Autodesk Inventor part; units mm, degrees
ref_plane "YZ Plane" through (0, 0, 0) normal (1, 0, 0) x (0, 1, 0)
ref_plane "XZ Plane" through (0, 0, 0) normal (0, 1, 0) x (-1, 0, 0)
ref_plane "XY Plane" through (0, 0, 0) normal (0, 0, 1) x (1, 0, 0)
sketch "Sketch1" plane through (0, 0, 0) normal (0, 0, 1) x (1, 0, 0)
  circle A0 centre (0, 0) radius 38
  circle A1 centre (0, 0) radius 33
  dimension "d0" = 76
  dimension "d1" = 66
extrude "Extrusion1" add sketch "Sketch1" along normal blind 15
sketch "Sketch2" plane through (0, 0, 0) normal (0, 0, -1) x (-1, 0, 0)
  circle A0 centre (0, 0) radius 33
  line L0 (0.0152, 1) -> (-32.9848, 1)
  line L1 (0.0152, -1) -> (-32.9848, -1)
  line L2 (0.0152, 1) -> (-12.0152, 1)
  circle A1 centre (0, 0) radius 33
  line L3 (0.0152, -1) -> (0.0152, 1)
  line L4 (-1, 0.0152) -> (-1, -32.9848)
  line L5 (1, 0.0152) -> (1, -32.9848)
  line L6 (-0.0152, -1) -> (32.9848, -1)
  line L7 (-0.0152, 1) -> (32.9848, 1)
  line L8 (1, -0.0152) -> (1, 32.9848)
  line L9 (-1, -0.0152) -> (-1, 32.9848)
  point P0 (-1, 1)
  point P1 (-1, -1)
  point P2 (1, -1)
  point P3 (1, 1)
  dimension "d12" = 2
  dimension "d17" = 66
  dimension "d18" = 33
  dimension "d19" = 33
  dimension "d22" = 360
extrude "Extrusion2" add sketch "Sketch2" against normal blind 15 contours A0 L6 L5 L8 L7 | L8 L7 L0 L9 A0 | L8 L5 L6 L3 L7 | A0 L4 L1 L6 L5 | L3 L1 L4 L9 L0 | L0 L9 L4 L1 A0
sketch "Sketch3" plane through (0, 0, 0) normal (0, 0, -1) x (-1, 0, 0)
  line L0 (0, 20) -> (-0.5, 20)
  line L1 (-0.5, 20) -> (-0.5, -20)
  line L2 (-0.5, -20) -> (0.5, -20)
  line L3 (0.5, -20) -> (0.5, 20)
  line L4 (0.5, 20) -> (0, 20)
  point P0 (0, 0)
  dimension "d27" = 20
  dimension "d29" = 40
  dimension "d30" = 1
  dimension "d31" = 40
extrude "Extrusion3" cut sketch "Sketch3" against normal blind 2
sketch "Sketch4" plane through (-1, 1, 0) normal (-1, 0, 0) x (0, 0, 1)
  point P0 (0, -1)
  point P1 (1.0253, 17.9677)
hole "Hole1" at (-1, 18.9677, 1.0253) direction (1, 0, 0) diameter 0.7 end through all
sketch "Sketch5" plane through (-1, -32.9848, 0) normal (-1, 0, 0) x (0, 0, 1)
  point P0 (0, 32.9848)
  point P1 (1.4149, 14.4794)
hole "Hole2" at (-1, -18.5055, 1.4149) direction (1, 0, 0) diameter 0.7 end through all
properties part number "SUJETADOR_MICRO"
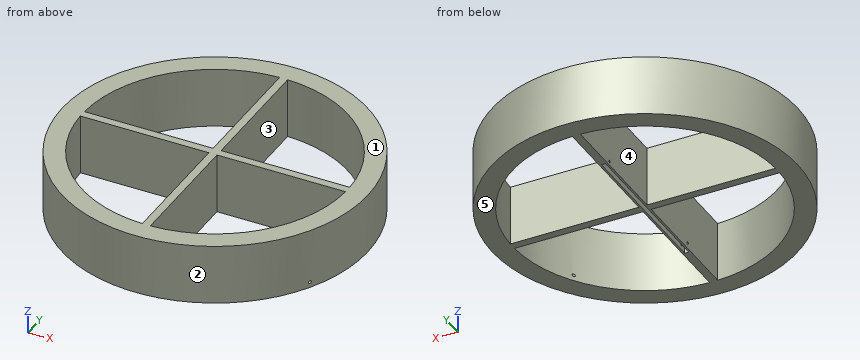
The listing builds one solid part. Answer for the finished solid, in the listing's coordinates (mm). Face numbers are marked on the shaded views. A direction names the side the tool comes from. Round coordinates to 2 decimals unless told otherwise and drop trailing zeros. Write each loop counter-clockwise with the first axis right and the second up, starting at its lowest first coordinate (ties: lowest second). Pieces come first, ordered by that corner, then holes. Notation, with made-up numbers: M -5.5,62 L 6.5,62 A22 ccw 6.5,87 Z; hole C 4.25,37.5 d2. An arc over 180 degrees is marked long. Write each question's results on one line, items separated by ' | '. Start each with the question number.
Item 1: Find section A-A on y = 30. Write down the section's boundary in (x, z).
Item 2: Find section C-C on z = 8.5. Write down the section's boundary in (x, y).
Item 3: Straight lines are drawn through the part: probe 1 along X at (y, z) = (-6, 11); probe 2 along X at (y, z) = (-12, 10). For each, find the intervals that lie inside material, in ascending order.
Item 4: Which of the six approach directions +Z, -Z, +X, -X, +Y, -Y give full straight-line access (tool end or side, diameter ignored) to the marked faces 4 and 5?
Item 5: The mould has two halves that part along X. Classify the marked faces 1, 2 and 3: +X half, -X half, draft (parallel to the pull), parting line (faces both ways), or undercut.
Item 6: Find section B-B on x = 9. Write down the section's boundary in (y, z), and give its area (3 significant figures).
Item 7: Given pin 1 Ø1 at (x, y) = (-26.5, 23.5) entering from -Z; pin 2 Ø8 at (x, z) = (-29.5, 10) entering from -Y; pin 3 Ø7.5 at (x, z) = (-17.5, 4.5) entering from -Y; pin 4 Ø0.5 at (x, z) = (0, 1) entering from -Y, each flat-ended and moving along its own axis, determine where each tip first touches the part or whether it passes through.
Answer block:
1) outline: M -23.32,0 L -13.75,0 L -13.75,15 L -23.32,15 Z; M -1,0 L 1,0 L 1,15 L -1,15 Z; M 13.75,0 L 23.32,0 L 23.32,15 L 13.75,15 Z
2) outline: C 0,0 d76; hole M -32.98,-1 A33 ccw -1,-32.98 L -1,-1 Z; hole M -32.98,1 L -1,1 L -1,32.98 A33 ccw Z; hole M 1,-32.98 A33 ccw 32.98,-1 L 1,-1 Z; hole M 1,1 L 32.98,1 A33 ccw 1,32.98 Z
3) probe 1: x = -37.52 to -32.45, -1 to 1, 32.45 to 37.52 | probe 2: x = -36.06 to -30.74, -1 to 1, 30.74 to 36.06
4) face 4: +Z, -Z | face 5: -Z, +X, -X, +Y, -Y
5) face 1: draft | face 2: parting line | face 3: undercut
6) outline: M -36.92,0 L -31.75,0 L -31.75,15 L -36.92,15 Z; M -1,0 L 1,0 L 1,15 L -1,15 Z; M 31.75,0 L 36.92,0 L 36.92,15 L 31.75,15 Z | area: 185 mm²
7) pin 1: stops at z = 0 | pin 2: stops at y = -28.17 | pin 3: stops at y = -35.43 | pin 4: stops at y = -38
